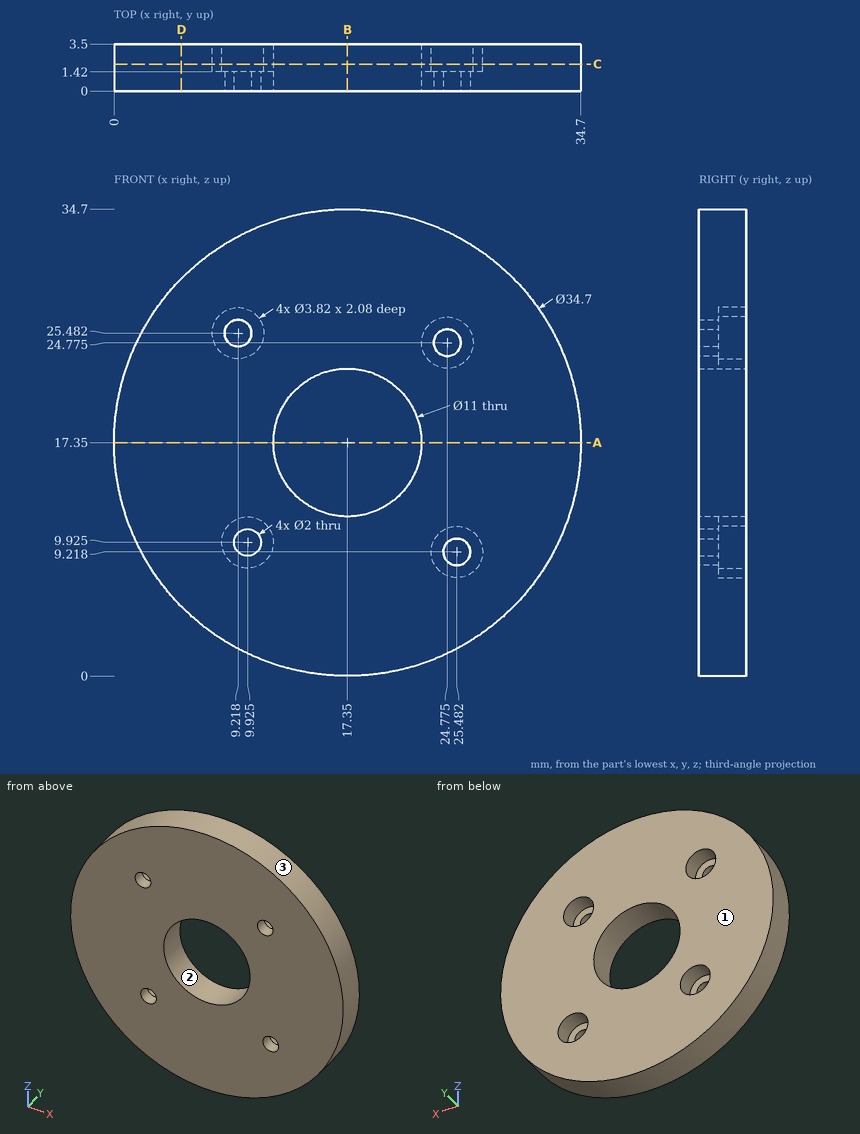
Geometry check sheet. Reference: drawing and pictorial views, mm from the part's lowest x, y, z. Round coordinates to 2 decimals unless told otherwise and drop trailing zeros. Loops run counter-clockwise (first coordinate to the right, second up) from the corner with the lowest first, then second, coordinate; pieces in that order, holes last. Notation, with made-up numbers: (-17, 13.5) - (18, 13.5) arc R28 cw to (18, 36.5) - close; hole circle Ø5 at (51.5, 49). An arc over 180 degrees is marked (long way). One line per question, with ' | ' between items. Start each with the question number.
1. Cross-section at B-B on x = 17.35. Record the cut outline in (y, z).
2. Depth check by flat-ended pin: pin 1 (1.5 mm diameter, centred on x = 19.5, y = 2, fed in from -Z); pin 2 (2 mm diameter, centred on y = 0.5, z = 24, fed in from -X) (1 decimal); pin 3 (1.1 mm diameter, centred on x = 24.5, z = 25.5, fed in from +Y). Enter the tip coordinate at first touch or a pass-through.
3. Scan lines: line 1 (X direction, y = 1.3, z = 17.35); line 2 (X direction, y = 2.25, z = 20) (1 decimal); line 3 (Z direction, x = 13, y = 0.75) (1 decimal). Record each from-to range of solid material in increasing order. Write a range as [from, to].
4. Cross-section at C-C on y = 2. State how many separate pieces and enclosed holes the cut face has, then the cut area to 3 significant figures.
5. Cross-section at D-D on x = 5. Record the cut outline in (y, z), then the cut area to 3 significant figures.
6. Draft check along Z on the marked faces 1, 2 and 3. Enter one of: released by +Z, released by -Z, zero draft, split by the parting line, or undercut.
7. Cross-section at A-A on z = 17.35. Record the cut outline in (x, y).
Taken from the geometry:
1) outline: (0, 0) - (3.5, 0) - (3.5, 11.85) - (0, 11.85) - close; (0, 22.85) - (3.5, 22.85) - (3.5, 34.7) - (0, 34.7) - close
2) pin 1: z = 0.06 | pin 2: x = 0.9 | pin 3: y = 1.42
3) line 1: [0, 11.85], [22.85, 34.7] | line 2: [0.2, 12.5], [22.2, 34.5] | line 3: [0.6, 14], [20.7, 34.1]
4) separate pieces: 1 | enclosed holes: 5 | area: 805 mm²
5) outline: (0, 5.16) - (3.5, 5.16) - (3.5, 29.54) - (0, 29.54) - close | area: 85.3 mm²
6) face 1: zero draft | face 2: undercut | face 3: split by the parting line
7) outline: (0, 0) - (11.85, 0) - (11.85, 3.5) - (0, 3.5) - close; (22.85, 0) - (34.7, 0) - (34.7, 3.5) - (22.85, 3.5) - close
